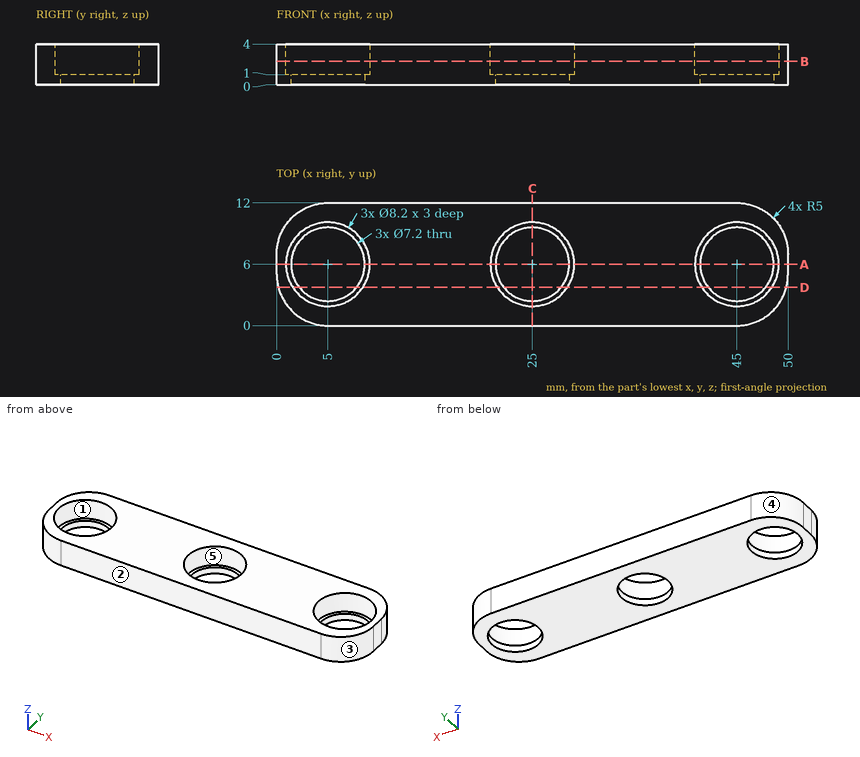
Check sheet for the drawn part. Datum: minimum x, y, z corner. Units: mm. A direction names the side the tool comes from. Round coordinates to 2 decimals unless told otherwise and drop trailing zeros. Loops run counter-clockwise (first coordinate to the right, second up) from the corner with the lowest first, then second, coordinate; pieces in that order, holes last. Notation, with made-up numbers: (-34, 64.5) - (21, 64.5) arc R34 ccw to (21, 95.5) - close; hole circle Ø10 at (68, 88.5). An arc over 180 degrees is marked (long way). Answer as a JSON object with one key per item and string values. Group by question number.
Q1. Sectioned sample at A-A, the plane y = 6. Enter the section's corners in (x, z).
Q2. Mould release check, pull along X, two halves, no side actions. Record for the marked faces 3, 4 and 5: released by +X, released by -X, zero draft, split by the parting line, or undercut.
Q3. Sectioned sample at D-D, the plane y = 3.75. Enter the section's corners in (x, z).
Q4. Gauge pin test, flat ends, axial feed: P1, Ø6.5, axis at x = 45.5, y = 6, coming from the +Z side; P2, Ø4.5, axis at x = 5, y = 6, coming from the +Z side; P3, Ø2, axis at y = 3, z = 1, coming from the -X side; P4, Ø1, axis at y = 9.5, z = 0.5, coming from the -X side. Record the tip position at first contact, or that the pin passes through.
Q5. Sectioned sample at B-B, the plane z = 2.3. Enter the section's corners in (x, y).
Q6. Sectioned sample at C-C, the plane x = 25. Enter the section's corners in (y, z).
Q7. Set-up check for the marked faces 1 and 2: record each of +Z, -Z, +X, -X, +Y, -Y from which the full face is reachable in a straight line by a thin tool's end or side.
Q8. Scan lines: line 1 along X through (y, z) = (3, 2.5); line 2 along Y through (x, z) = (25, 3.1); line 3 along Y through (x, z) = (5, 0.65). Record each from-to range of solid material in increasing order. Write a range as [from, to].
Solution:
{
 "1": {"outline": "(0, 0) - (1.4, 0) - (1.4, 1) - (0.9, 1) - (0.9, 4) - (0, 4) - close; (8.6, 0) - (21.4, 0) - (21.4, 1) - (20.9, 1) - (20.9, 4) - (9.1, 4) - (9.1, 1) - (8.6, 1) - close; (28.6, 0) - (41.4, 0) - (41.4, 1) - (40.9, 1) - (40.9, 4) - (29.1, 4) - (29.1, 1) - (28.6, 1) - close; (48.6, 0) - (50, 0) - (50, 4) - (49.1, 4) - (49.1, 1) - (48.6, 1) - close"},
 "2": {"face 3": "released by +X", "face 4": "released by -X", "face 5": "undercut"},
 "3": {"outline": "(0.16, 0) - (2.19, 0) - (2.19, 1) - (1.57, 1) - (1.57, 4) - (0.16, 4) - close; (7.81, 0) - (22.19, 0) - (22.19, 1) - (21.57, 1) - (21.57, 4) - (8.43, 4) - (8.43, 1) - (7.81, 1) - close; (27.81, 0) - (42.19, 0) - (42.19, 1) - (41.57, 1) - (41.57, 4) - (28.43, 4) - (28.43, 1) - (27.81, 1) - close; (47.81, 0) - (49.84, 0) - (49.84, 4) - (48.43, 4) - (48.43, 1) - (47.81, 1) - close"},
 "4": {"P1": "stops at z = 1", "P2": "passes through", "P3": "stops at x = 0.1", "P4": "stops at x = 0.42"},
 "5": {"outline": "(0, 5) arc R5 ccw to (5, 0) - (45, 0) arc R5 ccw to (50, 5) - (50, 7) arc R5 ccw to (45, 12) - (5, 12) arc R5 ccw to (0, 7) - close; hole circle Ø8.2 at (5, 6); hole circle Ø8.2 at (25, 6); hole circle Ø8.2 at (45, 6)"},
 "6": {"outline": "(0, 0) - (2.4, 0) - (2.4, 1) - (1.9, 1) - (1.9, 4) - (0, 4) - close; (9.6, 0) - (12, 0) - (12, 4) - (10.1, 4) - (10.1, 1) - (9.6, 1) - close"},
 "7": {"face 1": "+Z", "face 2": "+Z, -Z, +X, -X, -Y"},
 "8": {"line 1": "x = [0.42, 2.21], [7.79, 22.21], [27.79, 42.21], [47.79, 49.58]", "line 2": "y = [0, 1.9], [10.1, 12]", "line 3": "y = [0, 2.4], [9.6, 12]"}
}
